Can you work these out from the model? Positions are in its coordinate system, mm. Coordinates: 2 decimals unless noted, no trailing zeros. Order: outer loops, then holes, each group sorted by start corner. A loop starts at its lowest first (then second) coordinate and runs counter-clockwise, first axis right, second up.
Autodesk Inventor part; units mm, degrees
ref_plane "YZ Plane" through (0, 0, 0) normal (1, 0, 0) x (0, 1, 0)
ref_plane "XZ Plane" through (0, 0, 0) normal (0, 1, 0) x (-1, 0, 0)
ref_plane "XY Plane" through (0, 0, 0) normal (0, 0, 1) x (1, 0, 0)
sketch "Sketch2" plane through (0, 0, 0) normal (0, 1, 0) x (-1, 0, 0)
  circle A0 centre (3, 0) radius 1.5
  circle A1 centre (3, 0) radius 3
  circle A2 centre (3, -10) radius 1.5
  circle A3 centre (3, -10) radius 3
  line L0 (6, 0) -> (6, -10)
  line L1 (0, -10) -> (0, 0)
  dimension "d40" = 6
  dimension "d39" = 3
  dimension "d41" = 3
  dimension "d42" = 6
extrude "Extrusion6" add sketch "Sketch2" along normal blind 1 contours A1 | L0 A3 L1 A1
extrude "Extrusion7" add sketch "Sketch2" along normal blind 2 contours A3
thread "Thread1"
properties part number "linkToActuator5"
1. Thinking about a two-plate mould opening in X: for faces 1 (the cylindrical face through (-3, 1, -13)), 2 (the flat face through (-3, 0, -5)), 3 (the cylindrical face through (-2.675, 0.986, -8.536)), which applies, pulls with the +X half, pulls with the -X half, needs draft (parallel to the pull), parting line crosses it, or undercut?
Completed:
face 1: parting line crosses it
face 2: needs draft
face 3: undercut
2. Imagine slicing it at A-A on x = -3. Please give me the cut outline in (y, z), then the cut area to 3 significant figures.
Completed:
outline: (0, -13) - (2, -13) - (2, -11.5) - (0, -11.5) - close; (0, -8.5) - (2, -8.5) - (2, -7) - (1, -7) - (1, -1.5) - (0, -1.5) - close; (0, 1.5) - (1, 1.5) - (1, 3) - (0, 3) - close
area: 13.0 mm2
3. Imagine slicing it at D-D on x = -1.2. Please give me the cut outline in (y, z).
Completed:
outline: (0, -12.4) - (2, -12.4) - (2, -7.6) - (1, -7.6) - (1, 2.4) - (0, 2.4) - close
4. Please list where these lines run through material, in increasing order: probe 1 along Z at (x, y) = (-3, 0.6); probe 2 along Z at (x, y) = (-4.25, 0.35); probe 3 along Y at (x, z) = (-0.95, -4).
Completed:
probe 1: z = -13 to -11.5, -8.5 to -1.5, 1.5 to 3
probe 2: z = -12.73 to -10.83, -9.17 to -0.83, 0.83 to 2.73
probe 3: y = 0 to 1
5. Imagine slicing it at B-B on z = -11. Please give me the cut outline in (x, y), then the cut area to 3 significant figures.
Completed:
outline: (-5.83, 0) - (-4.12, 0) - (-4.12, 2) - (-5.83, 2) - close; (-1.88, 0) - (-0.17, 0) - (-0.17, 2) - (-1.88, 2) - close
area: 6.84 mm2
6. I'm going to push flat-ended pins straight in: pin 1 (2.5 mm diameter, centred on x = -3, z = 0, fed in from -Y); pin 2 (1.5 mm diameter, centred on x = -2, z = -4.5, fed in from +Y). Where does each tip first touch, or does it pass through?
Completed:
pin 1: passes through
pin 2: stops at y = 1
7. Imagine slicing it at C-C on y = 0.75. Please give me the cut outline in (x, z), then the cut area to 3 significant figures.
Completed:
outline: (-6, -10) arc R3 ccw to (0, -10) - (0, 0) arc R3 ccw to (-6, 0) - close; hole circle Ø3 at (-3, -10); hole circle Ø3 at (-3, 0)
area: 74.1 mm2
